Source: three-view drawing plus pictorial views. Frame: mm from the lowest corner of the part. A direction names the side the tool comes from. Give positions to 0.01 mm unless a question says otherwise; leave off trailing zeros. Order: outer loops, then holes, each group sorted by start corner. A loop starts at its lowest first (then second) coordinate and runs counter-clockwise, first axis right, second up. Notation, with made-up numbers: (81, 31) - (128, 31) arc R23 cw to (128, 65) - close; hole circle Ø4 at (63, 66.25). An arc over 180 degrees is marked (long way). Answer in a Markdown table with one row per item. Add a question column.
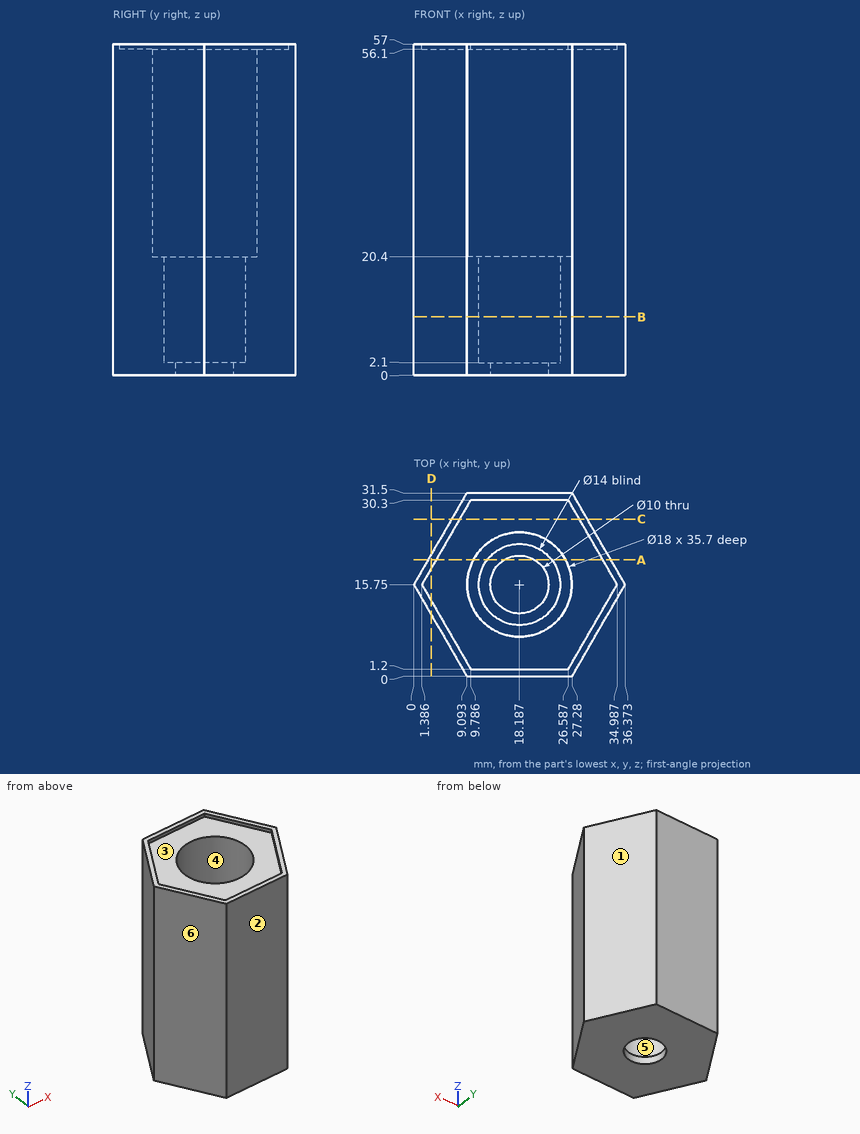
Q1. Section A-A, the plane y = 20. Return loops of the section in (x, z) (1 decimal).
Q2. Line query: probe 1 along Z at (x, y) = (30.5, 19); probe 2 along X at (y, z) = (15.75, 45) (1 decimal); probe 3 along Y at (x, z) = (26, 54) (1 decimal). Output: solid intervals per line, ascending.
Q3. Section B-B, the plane z = 10. Return loops of the section in (x, y).
Q4. Pull-direction query (Y, two-part tool) for the marked faces 1, 2, 3 and 4; classes: +Y half, -Y half, draft (parallel to the pull), parting line (faces both ways), or undercut.
Q5. Contact query for flat-ended pins moving along their axis: P1, Ø11, axis at x = 18.19, y = 15.75, coming from the +Z side; P2, Ø3, axis at y = 21.5, z = 50, coming from the +X side; P3, Ø8, axis at x = 18.19, y = 15.75, coming from the +Z side; P4, Ø0.7, axis at x = 18.5, z = 56.5, coming from the -Y side. Output: stop coordinate, or through.
Q6. Access query for the marked faces 5 and 6. Directions: +Z, -Z, +X, -X, +Y, -Y. A direction counts if a zero-diameter tool reaches every point of the face in a straight line with its end or side. Return the directions, or none.
Q7. Section D-D, the plane x = 3. Return loops of the section in (y, z), then the cut area to 3 significant figures.
Q8. Section C-C, the plane y = 27. Return loops of the section in (x, z) (1 decimal), then the cut area to 3 significant figures.
Computed:
| question | item | result |
|---|---|---|
| 1 | outline | (2.5, 0) - (15.6, 0) - (15.6, 2.1) - (12.6, 2.1) - (12.6, 20.4) - (10.3, 20.4) - (10.3, 56.1) - (3.8, 56.1) - (3.8, 57) - (2.5, 57) - close; (20.8, 0) - (33.9, 0) - (33.9, 57) - (32.5, 57) - (32.5, 56.1) - (26.1, 56.1) - (26.1, 20.4) - (23.7, 20.4) - (23.7, 2.1) - (20.8, 2.1) - close |
| 2 | probe 1 | z = 0 to 56.1 |
| 2 | probe 2 | x = 0 to 9.2, 27.2 to 36.4 |
| 2 | probe 3 | y = 0 to 11.3, 20.2 to 31.5 |
| 3 | outline | (0, 15.75) - (9.09, 0) - (27.28, 0) - (36.37, 15.75) - (27.28, 31.5) - (9.09, 31.5) - close; hole circle Ø14 at (18.19, 15.75) |
| 4 | face 1 | +Y half |
| 4 | face 2 | -Y half |
| 4 | face 3 | undercut |
| 4 | face 4 | undercut |
| 5 | P1 | stops at z = 2.1 |
| 5 | P2 | stops at x = 33.92 |
| 5 | P3 | passes through |
| 5 | P4 | stops at y = 0 |
| 6 | face 5 | +Z |
| 6 | face 6 | +Z, -Z, -X, -Y |
| 7 | outline | (10.55, 0) - (20.95, 0) - (20.95, 57) - (18.55, 57) - (18.55, 56.1) - (12.95, 56.1) - (12.95, 57) - (10.55, 57) - close |
| 7 | area | 587 mm^2 |
| 8 | outline | (6.5, 0) - (29.9, 0) - (29.9, 57) - (28.5, 57) - (28.5, 56.1) - (7.9, 56.1) - (7.9, 57) - (6.5, 57) - close |
| 8 | area | 1,310 mm^2 |
